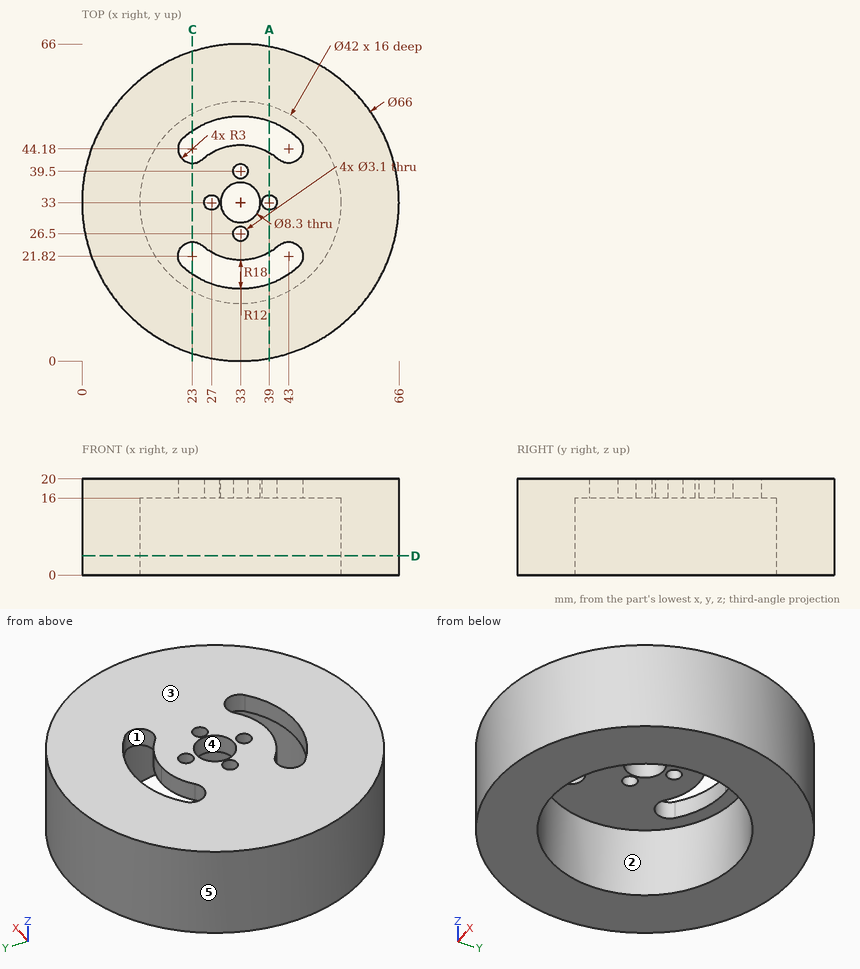
Verification items for this drawing (mm, ordinates from the low corner). A direction names the side the tool comes from. Coordinates: 2 decimals unless noted, no trailing zeros. Loops run counter-clockwise (first coordinate to the right, second up) from the corner with the lowest first, then second, coordinate; pieces in that order, holes last.
Item 1: Sectioned sample at A-A, the plane x = 39. Count the separate pieces of the cut face and the enclosed holes in it, then the cut area to 3 significant figures.
Item 2: Go/stop test with flat-tipped pins: pin 1 Ø5 at (y, z) = (36, 3) entering from +X; pin 2 Ø1.5 at (y, z) = (7.5, 6.5) entering from +X; pin 3 Ø21 at (x, y) = (29, 41) entering from -Z; pin 4 Ø1.9 at (x, y) = (27, 33) entering from +Z. Record where each tip stops, or that it passes through.
Item 3: Release check for a two-part mould opening along Y. For the marked faces 3, 4 and 5 record: released by +Y, released by -Y, zero draft, split by the parting line, or undercut.
Item 4: Thickness scan on line 1 (Y direction, x = 39, z = 16.8); line 2 (Y direction, x = 21.5, z = 8.5); line 3 (X direction, y = 39.5, z = 18.8). Record the ranges inside material, lowest first.
Item 5: Access from +Z, -Z, +X, -X, +Y, -Y to the whole of each face (thin tool, end or side, straight path). Record for the marked faces 1 and 2.
Item 6: Sectioned sample at C-C, the plane x = 23. Record the boundary of the cut face in (y, z).
Item 7: Sectioned sample at D-D, the plane z = 4. Record the boundary of the cut face in (x, y), then the cut area to 3 significant figures.
Check result:
1. separate pieces: 4
1. enclosed holes: 0
1. area: 589 mm2
2. pin 1: stops at x = 66
2. pin 2: stops at x = 54.83
2. pin 3: stops at z = 16
2. pin 4: passes through
3. face 3: zero draft
3. face 4: undercut
3. face 5: split by the parting line
4. line 1: y = 0.55 to 16.03, 22.61 to 31.45, 34.55 to 43.39, 49.97 to 65.45
4. line 2: y = 2.07 to 15.43, 50.57 to 63.93
4. line 3: x = 0.65 to 31.45, 34.55 to 65.35
5. face 1: +Z, -Z
5. face 2: -Z
6. outline: (1.55, 0) - (14.53, 0) - (14.53, 16) - (18.03, 16) - (18.03, 20) - (1.55, 20) - close; (24.82, 16) - (41.18, 16) - (41.18, 20) - (24.82, 20) - close; (47.97, 16) - (51.47, 16) - (51.47, 0) - (64.45, 0) - (64.45, 20) - (47.97, 20) - close
7. outline: circle Ø66 at (33, 33); hole circle Ø42 at (33, 33)
7. area: 2,040 mm2
